The model under review builds one solid part; all positions refer to its coordinate system, in mm. Face numbers are marked on the shaded views. A direction names the side the tool comes from. Round coordinates to 2 decimals unless told otherwise and drop trailing zeros. Order: outer loops, then holes, each group sorted by start corner. A loop starts at its lowest first (then second) coordinate and runs counter-clockwise, first axis right, second up. Notation, with made-up numbers: (1, 88.25) -> (24, 88.25) arc R17 ccw to (24, 111.25) -> close; hole circle Ø1 at (34, 56.5). An arc over 180 degrees is marked (long way). Return JSON: item names as keys, results as strings. Group by question number.
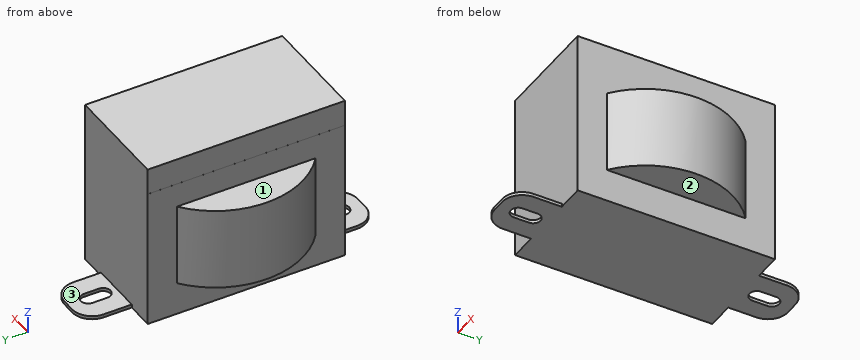
from build123d import *

# Parameters (mm, degrees)
SKETCH_1_W      = 32.5
SKETCH_1_H      = 59.5
EXTRUDE_1_DEPTH = 42.4
EXTRUDE_2_DEPTH = 25
EXTRUDE_3_DEPTH = 1
SKETCH_5_W      = 32.493243018
SKETCH_5_H      = 59.5
EXTRUDE_5_DEPTH = 8


with BuildPart() as part:
    # 草图1 → 拉伸1 (new body)
    with BuildSketch(Plane.XY):
        Rectangle(SKETCH_1_W, SKETCH_1_H)
    extrude(amount=EXTRUDE_1_DEPTH)

    # 草图2 → 拉伸2 (add)
    with BuildSketch(Plane.XY.offset(10)):
        with BuildLine():
            Line((-16.25, 20.932928605), (16.25, 20.932928605))
            ThreePointArc((16.25, 20.932928605), (26.5, 0), (16.25, -20.932928605))
            Line((16.25, -20.932928605), (-16.25, -20.932928605))
            ThreePointArc((-16.25, -20.932928605), (-26.5, 0), (-16.25, 20.932928605))
        make_face()
    extrude(amount=EXTRUDE_2_DEPTH)

    # 草图4 → 拉伸3 (add)
    # profile 1 of 2: a face of its own
    with BuildSketch(Plane.XY):
        with BuildLine():
            Line((-2, 44.25), (2, 44.25))
            ThreePointArc((2, 44.25), (6.242640687, 42.492640687), (8, 38.25))
            Line((8, 38.25), (8, 29.75))
            Line((8, 29.75), (-8, 29.75))
            Line((-8, 29.75), (-8, 38.25))
            ThreePointArc((-8, 38.25), (-6.242640687, 42.492640687), (-2, 44.25))
        make_face()
        with BuildLine():
            Line((-2.25, 38.25), (-2.25, 33.75))
            ThreePointArc((-2.25, 33.75), (0, 31.5), (2.25, 33.75))
            Line((2.25, 33.75), (2.25, 38.25))
            ThreePointArc((2.25, 38.25), (0, 40.5), (-2.25, 38.25))
        make_face(mode=Mode.SUBTRACT)
    # profile 2 of 2: a face of its own
    with BuildSketch(Plane.XY):
        with BuildLine():
            Line((-2, -44.25), (2, -44.25))
            ThreePointArc((2, -44.25), (6.242640687, -42.492640687), (8, -38.25))
            Line((8, -38.25), (8, -29.75))
            Line((8, -29.75), (-8, -29.75))
            Line((-8, -29.75), (-8, -38.25))
            ThreePointArc((-8, -38.25), (-6.242640687, -42.492640687), (-2, -44.25))
        make_face()
        with BuildLine():
            Line((2.25, -38.25), (2.25, -33.75))
            ThreePointArc((2.25, -33.75), (0, -31.5), (-2.25, -33.75))
            Line((-2.25, -33.75), (-2.25, -38.25))
            ThreePointArc((-2.25, -38.25), (0, -40.5), (2.25, -38.25))
        make_face(mode=Mode.SUBTRACT)
    extrude(amount=EXTRUDE_3_DEPTH)

    # 草图5 → 拉伸5 (add)
    with BuildSketch(Plane.XY.offset(42.4)):
        with Locations((0.003378491, 0)):
            Rectangle(SKETCH_5_W, SKETCH_5_H)
    extrude(amount=EXTRUDE_5_DEPTH)


solid = part.part
Item 1: Consider section B-B on z = 14. State the section outline as (x, y) points, plus the area to 3 significant figures.
Item 2: Consider section D-D on x = 9. State the section outline as (y, z) points.
Item 3: Insertion check: pin 1 Ø1.1 at (y, z) = (-32.5, 0.5) entering from +X; pin 2 Ø12 at (x, y) = (13.5, -15) entering from -Z; pin 3 Ø15 at (y, z) = (2, 34) entering from +X; pin 4 Ø1 at (x, z) = (-11, 39.5) entering from +Y. Each pin has a flat end and moves straight along its axis. Give the tip position at first contact, or say it passes through.
Item 4: For the marked faces 1, 2 and 3, list the 3-axis set-ups (+Z, -Z, +X, -X, +Y, -Y) from which the entire face can be reached by the end or side of a thin tool; tool diameter is ignored.
Item 5: Wall thickness on line 1 along Y through (x, z) = (-9.5, 29.5); line 2 along X through (y, z) = (-24, 33.5); line 3 along Z through (x, y) = (20, 7.5): over which ranges is each line inside the solid? List them lowest first.
Item 6: Consider section A-A on x = 0. State the section outline as (y, z) points.
Values:
{
 "1": {"outline": "(-16.25, -29.75) -> (16.25, -29.75) -> (16.25, -20.93) arc R26.5 ccw to (16.25, 20.93) -> (16.25, 29.75) -> (-16.25, 29.75) -> (-16.25, 20.93) arc R26.5 ccw to (-16.25, -20.93) -> close", "area": "2,530 mm^2"},
 "2": {"outline": "(-29.75, 0) -> (29.75, 0) -> (29.75, 50.4) -> (-29.75, 50.4) -> close"},
 "3": {"pin 1": "x = 8", "pin 2": "z = 0", "pin 3": "x = 26.5", "pin 4": "y = 29.75"},
 "4": {"face 1": "+Z, -X, +Y, -Y", "face 2": "-Z, +X, +Y, -Y", "face 3": "+Z, +X, -X, +Y"},
 "5": {"line 1": "-29.75 to 29.75", "line 2": "-16.25 to 16.25", "line 3": "10 to 35"},
 "6": {"outline": "(-44.25, 0) -> (-40.5, 0) -> (-40.5, 1) -> (-44.25, 1) -> close; (-31.5, 0) -> (31.5, 0) -> (31.5, 1) -> (29.75, 1) -> (29.75, 50.4) -> (-29.75, 50.4) -> (-29.75, 1) -> (-31.5, 1) -> close; (40.5, 0) -> (44.25, 0) -> (44.25, 1) -> (40.5, 1) -> close"}
}
